Autodesk Inventor part; units mm, degrees
ref_plane "YZ Plane" through (0, 0, 0) normal (1, 0, 0) x (0, 1, 0)
ref_plane "XZ Plane" through (0, 0, 0) normal (0, 1, 0) x (-1, 0, 0)
ref_plane "XY Plane" through (0, 0, 0) normal (0, 0, 1) x (1, 0, 0)
ref_plane "Work Plane1" through (0, 0, 6) normal (0, 0, 1) x (1, 0, 0)
sketch "Sketch2" plane through (0, 0, 6) normal (0, 0, 1) x (1, 0, 0)
  circle A0 centre (30, 51.3034) radius 1.5 construction
  circle A1 centre (30, 27.3034) radius 1.5 construction
  circle A2 centre (0, 51.3034) radius 1.5 construction
  circle A3 centre (0, 27.3034) radius 1.5 construction
  circle A4 centre (-30, 51.3034) radius 1.5 construction
  circle A5 centre (-30, 27.3034) radius 1.5 construction
  line L0 (36, 57.3034) -> (-36, 57.3034)
  line L1 (-36, 57.3034) -> (-36, 21.3034)
  line L2 (-36, 21.3034) -> (36, 21.3034)
  line L3 (36, 21.3034) -> (36, 57.3034)
  circle A6 centre (30, 51.3034) radius 1.9
  circle A7 centre (30, 27.3034) radius 1.9
  circle A8 centre (0, 51.3034) radius 1.9
  circle A9 centre (0, 27.3034) radius 1.9
  circle A10 centre (-30, 51.3034) radius 1.9
  circle A11 centre (-30, 27.3034) radius 1.9
  point P0 (0, 0)
  dimension "d0" = 6
  dimension "d1" = 6
  dimension "d2" = 6
  dimension "d3" = 6
  dimension "d4" = 0.4
  dimension "d5" = 0.4
  dimension "d6" = 0.4
  dimension "d7" = 0.4
  dimension "d8" = 0.4
  dimension "d9" = 0.4
extrude "Extrusion1" add sketch "Sketch2" along normal blind 1.75
fillet "Fillet1" radius 3 4 edges at (-36, 57.3034, 6.875) (-36, 21.3034, 6.875) (36, 57.3034, 6.875) (36, 21.3034, 6.875)
properties part number "Board"
Geometry: final body of the model. Coordinates: model frame, mm. Give positions to 0.01 mm unless a question says otherwise; leave off trailing zeros. Write each loop counter-clockwise with the first axis right and the second up, starting at its lowest first coordinate (ties: lowest second). Pieces come first, ordered by that corner, then holes.
1. Section query A-A, the plane x = 30. Return loops of the section in (y, z).
2. Draft query along Y for faces 1 (the cylindrical face through (35.145, 56.401, 6.887)), 2 (the cylindrical face through (-28.98, 25.7, 6.86)), 3 (the flat face through (-1, 40, 6)). Return one class per face: released by +Y, released by -Y, zero draft, split by the parting line, or undercut.
3. Pin query (flat end, axial travel): P1, Ø2.5, axis at x = 30, y = 51.3, coming from the +Z side (3 decimals). Return the tip coordinate at first contact, or that it passes through.
4. Line query: probe 1 along Y at (x, z) = (30, 6.65); probe 2 along X at (y, z) = (27, 6.3); probe 3 along X at (y, z) = (53, 6.55). Output: solid intervals per line, ascending.
5. Section query B-B, the plane z = 6.75. Return loops of the section in (x, y).
Computed:
1. outline: (21.3, 6) - (25.4, 6) - (25.4, 7.75) - (21.3, 7.75) - close; (29.2, 6) - (49.4, 6) - (49.4, 7.75) - (29.2, 7.75) - close; (53.2, 6) - (57.3, 6) - (57.3, 7.75) - (53.2, 7.75) - close
2. face 1: released by +Y
2. face 2: undercut
2. face 3: zero draft
3. P1: passes through
4. probe 1: y = 21.3 to 25.4, 29.2 to 49.4, 53.2 to 57.3
4. probe 2: x = -36 to -31.88, -28.12 to -1.88, 1.88 to 28.12, 31.88 to 36
4. probe 3: x = -36 to -30.86, -29.14 to -0.86, 0.86 to 29.14, 30.86 to 36
5. outline: (-36, 24.3) arc R3 ccw to (-33, 21.3) - (33, 21.3) arc R3 ccw to (36, 24.3) - (36, 54.3) arc R3 ccw to (33, 57.3) - (-33, 57.3) arc R3 ccw to (-36, 54.3) - close; hole circle Ø3.8 at (-30, 27.3); hole circle Ø3.8 at (-30, 51.3); hole circle Ø3.8 at (0, 27.3); hole circle Ø3.8 at (0, 51.3); hole circle Ø3.8 at (30, 27.3); hole circle Ø3.8 at (30, 51.3)
